Check sheet for the drawn part. Datum: minimum x, y, z corner. Units: mm. A direction names the side the tool comes from. Round coordinates to 2 decimals unless told otherwise and drop trailing zeros. Write each loop counter-clockwise with the first axis right and the second up, starting at its lowest first coordinate (ties: lowest second). Pieces come first, ordered by that corner, then holes. Notation, with made-up numbers: M 4,-40 L 30,-40 A13 cw 30,-22 Z; hole C 34.25,-26.75 d2. An arc over 180 degrees is marked long. One line per item, written item: value. Start each with the question number.
Item 1: Section check D-D, the plane x = 14.25. Record the cut outline in (y, z), then the cut area to 3 significant figures.
Item 2: Gauge pin test, flat ends, axial feed: pin 1 (5 mm diameter, centred on y = 6, z = 23.5, fed in from -X); pin 2 (4.5 mm diameter, centred on x = 5.1, z = 11.5, fed in from -Y); pin 3 (2 mm diameter, centred on x = 17, z = 26.5, fed in from +Y); pin 4 (2 mm diameter, centred on x = 12.5, y = 24.5, fed in from +Z). Record the tip position at first contact, or that the pin passes through.
Item 3: Section check C-C, the plane z = 18.5. Record the cut outline in (x, y).
Item 4: Thickness scan on probe 1 along X at (y, z) = (1.05, 25.5); probe 2 along Z at (x, y) = (5.1, 1.6); probe 3 along X at (y, z) = (20, 1). Record the ranges inside material, lowest first. Write a range as from..to.
Item 5: Draft check along X on the marked faces 3, 4 and 5. Enter one of: +X half, -X half, draft (parallel to the pull), parting line (faces both ways), or undercut.
Item 6: Section check A-A, the plane z = 25.5. Record the cut outline in (x, y).
Item 7: Section check B-B, the plane y = 21. Record the cut outline in (x, z).
Item 8: Tool access check on the marked faces 1 and 2. Record the directions out of +Z, -Z, +X, -X, +Y, -Y that give a thin tool (end or side, any length) a straight path to the whole face; none if there is none.
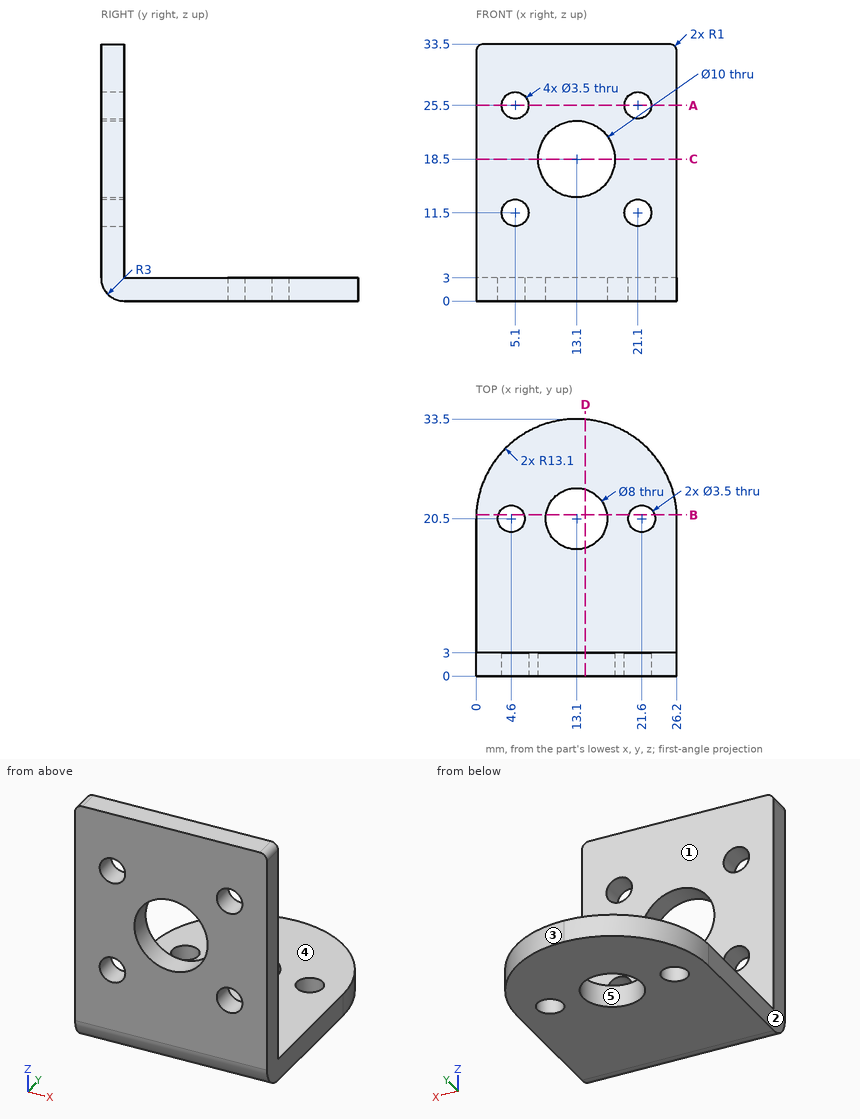
Response values:
1. outline: M 0,3 A3 ccw 3,0 L 16.67,0 L 16.67,3 L 3,3 L 3,13.63 L 0,13.63 Z; M 0,23.37 L 3,23.37 L 3,33.5 L 0,33.5 Z; M 24.33,0 L 33.45,0 L 33.45,3 L 24.33,3 Z
1. area: 138 mm2
2. pin 1: passes through
2. pin 2: stops at y = 0
2. pin 3: stops at y = 3
2. pin 4: stops at z = 3
3. outline: M 0,0 L 8.1,0 L 8.1,3 L 0,3 Z; M 18.1,0 L 26.2,0 L 26.2,3 L 18.1,3 Z
4. probe 1: x = 0..3.35, 6.85..19.35, 22.85..26.2
4. probe 2: z = 0.35..9.75, 13.25..23.75, 27.25..33.5
4. probe 3: x = 0..2.92, 6.28..9.13, 17.07..19.92, 23.28..26.2
5. face 3: +X half
5. face 4: draft
5. face 5: undercut
6. outline: M 0,0 L 3.35,0 L 3.35,3 L 0,3 Z; M 6.85,0 L 19.35,0 L 19.35,3 L 6.85,3 Z; M 22.85,0 L 26.2,0 L 26.2,3 L 22.85,3 Z
7. outline: M 0.01,0 L 2.92,0 L 2.92,3 L 0.01,3 Z; M 6.28,0 L 9.13,0 L 9.13,3 L 6.28,3 Z; M 17.07,0 L 19.92,0 L 19.92,3 L 17.07,3 Z; M 23.28,0 L 26.19,0 L 26.19,3 L 23.28,3 Z
8. face 1: +Z, +X, -X, +Y
8. face 2: +Z, -Z, -X, +Y, -Y
